from build123d import *

# Parameters (mm, degrees)
F1_DEPTH = 70
F2_W     = 20
F2_H     = 30
F3_DEPTH = 35.001
F5_DEPTH = 130.001


with BuildPart() as f1:
    # F0 (on Front) → F1 (new body)
    with BuildSketch(Plane.XZ):
        Polygon((-65, 0), (-65, -35), (65, -35), (65, 35), (15, 35), (-25, 0), align=None)
    extrude(amount=F1_DEPTH)

    # F2 (on face) → F3 (cut, through all)
    with BuildSketch(Plane.XY):
        with Locations((-55, -35)):
            Rectangle(F2_W, F2_H)
    extrude(amount=-F3_DEPTH, mode=Mode.SUBTRACT)

    # F4 (on face) → F5 (cut, through all)
    with BuildSketch(Plane.YZ.offset(65)):
        with BuildLine():
            ThreePointArc((-55, 10), (-53.535534, 6.464466), (-50, 5))
            Line((-50, 5), (-20, 5))
            ThreePointArc((-20, 5), (-16.464466, 6.464466), (-15, 10))
            Line((-15, 10), (-15, 20))
            ThreePointArc((-15, 20), (-16.464466, 23.535534), (-20, 25))
            Line((-20, 25), (-50, 25))
            ThreePointArc((-50, 25), (-53.535534, 23.535534), (-55, 20))
            Line((-55, 20), (-55, 10))
        make_face()
    extrude(amount=-F5_DEPTH, mode=Mode.SUBTRACT)


solid = f1.part
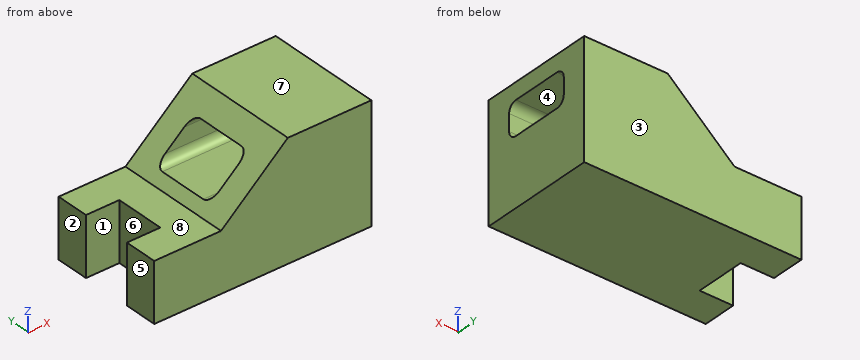
Work out the finished part from the listing and answer in its coordinate system (mm). Face numbers are marked on the shaded views. A direction names the side the tool comes from. Give positions to 0.01 mm unless a question says otherwise; leave off trailing zeros. Order: outer loops, then holes, each group sorted by start corner. A loop starts at its lowest first (then second) coordinate and runs counter-clockwise, first axis right, second up. Notation, with made-up numbers: (25.5, -11.5) -> (69.5, -11.5) arc R21 cw to (69.5, -4.5) -> close; hole circle Ø4 at (-37, -16.5). An arc over 180 degrees is marked (long way). Answer as a JSON object with one key per item and string values. Group by question number.
1. Section C-C on x = 33 is taken. Determine the outline of the cut face in (y, z).
2. A tool of negligible diameter and unlimited length cuts with its end or side. For the marked faces 4, 5, 6, 7 and 8, from which of +Z, -Z, +X, -X, +Y, -Y can it reach the whole face along a straight path? Write none if from no direction.
3. Section A-A on x = -49.5 is taken. Determine the outline of the cut face in (y, z), plus the area to 3 significant figures.
4. Consider line 1 along Y through (x, z) = (2.5, 10); line 2 along Z through (x, y) = (25.5, -23); line 3 along X through (y, z) = (-29, -22.5). Determine where each line is inside the solid, lowest interval first. Write a range as [from, to].
5. Section D-D on z = -10 is taken. Determine the outline of the cut face in (x, y).
6. Flat-ended cylindrical pins translate along their axes: pin 1 Ø9 at (y, z) = (-28.5, -21.5) entering from -X; pin 2 Ø4 at (y, z) = (-50.5, 4.5) entering from -X. Find the tip coordinate at first contact, or state that the pin passes through.
7. The mould has two halves that part along Y. Classify the marked faces 1, 2 and 3: released by +Y, released by -Y, zero draft, split by the parting line, or undercut.
8. Section B-B on y = -48 is taken. Determine the outline of the cut face in (x, z), plus the area to 3 significant figures.
Result sheet:
{
 "1": {"outline": "(-70, -35) -> (0, -35) -> (0, 35) -> (-70, 35) -> close; hole (-55, 10) arc R5 ccw to (-50, 5) -> (-20, 5) arc R5 ccw to (-15, 10) -> (-15, 20) arc R5 ccw to (-20, 25) -> (-50, 25) arc R5 ccw to (-55, 20) -> close"},
 "2": {"face 4": "+X, -X", "face 5": "+Z, -Z, -X, +Y, -Y", "face 6": "+Z, -Z, -X", "face 7": "+Z, +X, -X, +Y, -Y", "face 8": "+Z, -X, +Y, -Y"},
 "3": {"outline": "(-70, -35) -> (-50, -35) -> (-50, 0) -> (-70, 0) -> close; (-20, -35) -> (0, -35) -> (0, 0) -> (-20, 0) -> close", "area": "1,400 mm^2"},
 "4": {"line 1": "y = [-70, -55], [-15, 0]", "line 2": "z = [-35, 5], [25, 35]", "line 3": "x = [-45, 65]"},
 "5": {"outline": "(-65, -70) -> (65, -70) -> (65, 0) -> (-65, 0) -> (-65, -20) -> (-45, -20) -> (-45, -50) -> (-65, -50) -> close"},
 "6": {"pin 1": "stops at x = -45", "pin 2": "stops at x = -22.14"},
 "7": {"face 1": "undercut", "face 2": "zero draft", "face 3": "released by +Y"},
 "8": {"outline": "(-45, -35) -> (65, -35) -> (65, 5) -> (-19.29, 5) -> (-25, 0) -> (-45, 0) -> close; (3.57, 25) -> (65, 25) -> (65, 35) -> (15, 35) -> close", "area": "4,840 mm^2"}
}
